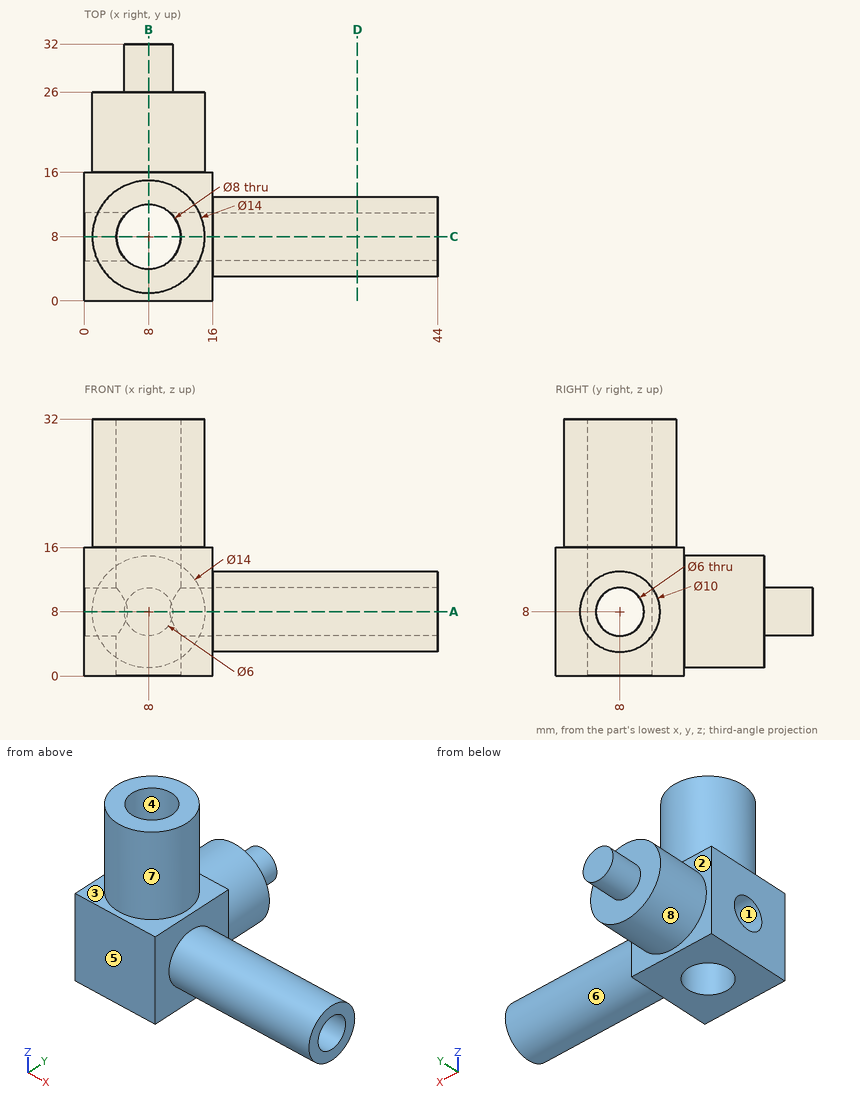
Study the drawing (mm; zero at the part's minimum x, y, z) and answer. A direction names the side the tool comes from. Give positions to 0.01 mm unless a question says otherwise; leave off trailing zeros. Write each loop counter-clockwise with the first axis right and the second up, starting at its lowest first coordinate (ties: lowest second). Pieces come first, ordered by that corner, then holes. Notation, with made-up numbers: (-28, -7.75) - (9, -7.75) arc R10 ccw to (9, 5.25) - close; hole circle Ø6 at (4, 56). An arc over 180 degrees is marked (long way). One line per question, with ' | ' between items. Start each with the question number.
1. Section D-D, the plane x = 34 is taken. Determine the outline of the cut face in (y, z), then the cut area to 3 significant figures.
2. Section B-B, the plane x = 8 is taken. Determine the outline of the cut face in (y, z), then the cut area to 3 significant figures.
3. Given P1, Ø6, axis at y = 22, z = 12, coming from the +X side; P2, Ø1, axis at y = 16.5, z = 28.5, coming from the +X side; P3, Ø1, axis at y = 6.5, z = 18.5, coming from the -X side; P4, Ø4, axis at x = 13.5, z = 4, coming from the +Y side, each flat-ended and moving along its own axis, determine where each tip first touches the part or whether it passes through.
4. Determine the mould class of the marked faces 1, 2, 3 and 4 for opening direction Y: +Y half, -Y half, draft (parallel to the pull), parting line (faces both ways), or undercut.
5. For the marked faces 5, 6, 7 and 8, determine the directions among +Z, -Z, +X, -X, +Y, -Y from which every point of the face is accessible in a straight line to the end or side of a thin tool.
6. Section A-A, the plane z = 8 is taken. Determine the outline of the cut face in (x, y).
7. Straight lines are drawn through the part: line 1 (Z direction, x = 13, y = 8); line 2 (Z direction, x = 30.75, y = 8); line 3 (Y direction, x = 8, z = 12). For each, find the intervals that lie inside material, in ascending order.
8. Section C-C, the plane y = 8 is taken. Determine the outline of the cut face in (x, z), then the cut area to 3 significant figures.
Result:
1) outline: circle Ø10 at (8, 8); hole circle Ø6 at (8, 8) | area: 50.3 mm2
2) outline: (0, 0) - (4, 0) - (4, 32) - (1, 32) - (1, 16) - (0, 16) - close; (12, 0) - (16, 0) - (16, 1) - (26, 1) - (26, 5) - (32, 5) - (32, 11) - (26, 11) - (26, 15) - (16, 15) - (16, 16) - (15, 16) - (15, 32) - (12, 32) - close | area: 400 mm2
3) P1: stops at x = 14.93 | P2: passes through | P3: stops at x = 1.07 | P4: stops at y = 26
4) face 1: undercut | face 2: +Y half | face 3: draft | face 4: undercut
5) face 5: +Z, -Z, +X, -X, -Y | face 6: +X | face 7: +Z | face 8: +Y
6) outline: (0, 0) - (16, 0) - (16, 3) - (44, 3) - (44, 5) - (10.65, 5) arc R4 cw to (5.35, 5) - (0, 5) - close; (0, 11) - (5.35, 11) arc R4 cw to (10.65, 11) - (44, 11) - (44, 13) - (16, 13) - (16, 16) - (15, 16) - (15, 26) - (11, 26) - (11, 32) - (5, 32) - (5, 26) - (1, 26) - (1, 16) - (0, 16) - close
7) line 1: z = 0 to 5, 11 to 32 | line 2: z = 3 to 5, 11 to 13 | line 3: y = 0 to 4, 12 to 26
8) outline: (0, 0) - (4, 0) - (4, 5) - (0, 5) - close; (0, 11) - (4, 11) - (4, 32) - (1, 32) - (1, 16) - (0, 16) - close; (12, 0) - (16, 0) - (16, 3) - (44, 3) - (44, 5) - (12, 5) - close; (12, 11) - (44, 11) - (44, 13) - (16, 13) - (16, 16) - (15, 16) - (15, 32) - (12, 32) - close | area: 288 mm2
